```python
from build123d import *

# Parameters (mm, degrees)
SKETCH1_R             = 1.9
BOSS_EXTRUDE1_DEPTH   = 2.8
SKETCH1_R_2           = 0.8
BOSS_EXTRUDE1_2_DEPTH = 2.8
BOSS_EXTRUDE1_3_DEPTH = 2.8
SKETCH1_R_3           = 0.6
BOSS_EXTRUDE1_4_DEPTH = 2.8
BOSS_EXTRUDE1_5_DEPTH = 2.8
SKETCH2_W             = 15.494
SKETCH2_H             = 15.494
BOSS_EXTRUDE2_DEPTH   = 11.1
BOSS_EXTRUDE3_DEPTH   = 3
CHAMFER1_SIZE         = 3
CHAMFER1_SIZE2        = 5.196152423
CHAMFER1_PART_2_SIZE  = 3
CHAMFER1_PART_2_SIZE2 = 5.196152423
CHAMFER1_PART_3_SIZE  = 3
CHAMFER1_PART_3_SIZE2 = 5.196152423
CHAMFER1_PART_4_SIZE  = 3
CHAMFER1_PART_4_SIZE2 = 5.196152423
CHAMFER2_SIZE         = 4
CHAMFER2_SIZE2        = 1.455880937
CHAMFER2_PART_2_SIZE  = 4
CHAMFER2_PART_2_SIZE2 = 1.455880937
CHAMFER2_PART_3_SIZE  = 4
CHAMFER2_PART_3_SIZE2 = 1.455880937
CHAMFER2_PART_4_SIZE  = 4
CHAMFER2_PART_4_SIZE2 = 1.455880937
CHAMFER3_SIZE         = 0.5


with BuildPart() as part:
    # Sketch1 → Boss-Extrude1 (new body)
    with BuildSketch(Plane(origin=(0, 0, 0), x_dir=(1, 0, 0), z_dir=(0, 1, 0))):
        Circle(SKETCH1_R)
    extrude(amount=-BOSS_EXTRUDE1_DEPTH)



with BuildPart() as body_2:
    # Sketch1 → Boss-Extrude1 2 (new body)
    with BuildSketch(Plane(origin=(0, 0, 0), x_dir=(1, 0, 0), z_dir=(0, 1, 0))):
        with Locations((5.08, 0)):
            Circle(SKETCH1_R_2)
    extrude(amount=-BOSS_EXTRUDE1_2_DEPTH)


with BuildPart() as body_3:
    # Sketch1 → Boss-Extrude1 3 (new body)
    with BuildSketch(Plane(origin=(0, 0, 0), x_dir=(1, 0, 0), z_dir=(0, 1, 0))):
        with Locations((-5.08, 0)):
            Circle(SKETCH1_R_2)
    extrude(amount=-BOSS_EXTRUDE1_3_DEPTH)


with BuildPart() as body_4:
    # Sketch1 → Boss-Extrude1 4 (new body)
    with BuildSketch(Plane(origin=(0, 0, 0), x_dir=(1, 0, 0), z_dir=(0, 1, 0))):
        with Locations((-3.81, 2.54)):
            Circle(SKETCH1_R_3)
    extrude(amount=-BOSS_EXTRUDE1_4_DEPTH)


with BuildPart() as body_5:
    # Sketch1 → Boss-Extrude1 5 (new body)
    with BuildSketch(Plane(origin=(0, 0, 0), x_dir=(1, 0, 0), z_dir=(0, 1, 0))):
        with Locations((2.54, 5.08)):
            Circle(SKETCH1_R_3)
    extrude(amount=-BOSS_EXTRUDE1_5_DEPTH)


with BuildPart() as part_1:
    add(part.part)

    add(body_2.part)  # Boss-Extrude2 merges body 2

    add(body_3.part)  # Boss-Extrude2 merges body 3

    add(body_4.part)  # Boss-Extrude2 merges body 4

    add(body_5.part)  # Boss-Extrude2 merges body 5
    # Sketch2 → Boss-Extrude2 (add)
    with BuildSketch(Plane(origin=(0, 0, 0), x_dir=(1, 0, 0), z_dir=(0, 1, 0))):
        Rectangle(SKETCH2_W, SKETCH2_H)
    extrude(amount=BOSS_EXTRUDE2_DEPTH)

    # Sketch3 → Boss-Extrude3 (add)
    with BuildSketch(Plane(origin=(0, 11.1, 0), x_dir=(-1, 0, 0), z_dir=(0, 1, 0))):
        Polygon((0.55, -2), (-0.55, -2), (-0.55, -0.55), (-2, -0.55), (-2, 0.55), (-0.55, 0.55), (-0.55, 2), (0.55, 2), (0.55, 0.55), (2, 0.55), (2, -0.55), (0.55, -0.55), align=None)
    extrude(amount=BOSS_EXTRUDE3_DEPTH)

    # Chamfer1
    chamfer1_edges = [part_1.edges().sort_by_distance(p)[0] for p in [
        (-7.747, 11.1, 0),
    ]]
    chamfer1_side = [part_1.faces().sort_by_distance(p)[0] for p in [
        (-7.747, 5.55, 0),
    ]]
    chamfer(chamfer1_edges, length=CHAMFER1_SIZE, length2=CHAMFER1_SIZE2, reference=chamfer1_side[0])

    # Chamfer1 part 2
    chamfer1_part_2_edges = [part_1.edges().sort_by_distance(p)[0] for p in [
        (0, 11.1, 7.747),
    ]]
    chamfer1_part_2_side = [part_1.faces().sort_by_distance(p)[0] for p in [
        (0, 5.55, 7.747),
    ]]
    chamfer(chamfer1_part_2_edges, length=CHAMFER1_PART_2_SIZE, length2=CHAMFER1_PART_2_SIZE2, reference=chamfer1_part_2_side[0])

    # Chamfer1 part 3
    chamfer1_part_3_edges = [part_1.edges().sort_by_distance(p)[0] for p in [
        (7.747, 11.1, 0),
    ]]
    chamfer1_part_3_side = [part_1.faces().sort_by_distance(p)[0] for p in [
        (7.747, 5.55, 0),
    ]]
    chamfer(chamfer1_part_3_edges, length=CHAMFER1_PART_3_SIZE, length2=CHAMFER1_PART_3_SIZE2, reference=chamfer1_part_3_side[0])

    # Chamfer1 part 4
    chamfer1_part_4_edges = [part_1.edges().sort_by_distance(p)[0] for p in [
        (0, 11.1, -7.747),
    ]]
    chamfer1_part_4_side = [part_1.faces().sort_by_distance(p)[0] for p in [
        (0, 5.55, -7.747),
    ]]
    chamfer(chamfer1_part_4_edges, length=CHAMFER1_PART_4_SIZE, length2=CHAMFER1_PART_4_SIZE2, reference=chamfer1_part_4_side[0])

    # Chamfer2
    chamfer2_edges = [part_1.edges().sort_by_distance(p)[0] for p in [
        (-7.747, 0, 0),
    ]]
    chamfer2_side = [part_1.faces().sort_by_distance(p)[0] for p in [
        (-7.747, 4.05, 0),
    ]]
    chamfer(chamfer2_edges, length=CHAMFER2_SIZE, length2=CHAMFER2_SIZE2, reference=chamfer2_side[0])

    # Chamfer2 part 2
    chamfer2_part_2_edges = [part_1.edges().sort_by_distance(p)[0] for p in [
        (0, 0, 7.747),
    ]]
    chamfer2_part_2_side = [part_1.faces().sort_by_distance(p)[0] for p in [
        (0, 4.05, 7.747),
    ]]
    chamfer(chamfer2_part_2_edges, length=CHAMFER2_PART_2_SIZE, length2=CHAMFER2_PART_2_SIZE2, reference=chamfer2_part_2_side[0])

    # Chamfer2 part 3
    chamfer2_part_3_edges = [part_1.edges().sort_by_distance(p)[0] for p in [
        (7.747, 0, 0),
    ]]
    chamfer2_part_3_side = [part_1.faces().sort_by_distance(p)[0] for p in [
        (7.747, 4.05, 0),
    ]]
    chamfer(chamfer2_part_3_edges, length=CHAMFER2_PART_3_SIZE, length2=CHAMFER2_PART_3_SIZE2, reference=chamfer2_part_3_side[0])

    # Chamfer2 part 4
    chamfer2_part_4_edges = [part_1.edges().sort_by_distance(p)[0] for p in [
        (0, 0, -7.747),
    ]]
    chamfer2_part_4_side = [part_1.faces().sort_by_distance(p)[0] for p in [
        (0, 4.05, -7.747),
    ]]
    chamfer(chamfer2_part_4_edges, length=CHAMFER2_PART_4_SIZE, length2=CHAMFER2_PART_4_SIZE2, reference=chamfer2_part_4_side[0])

    # Chamfer3
    chamfer3_edges = [part_1.edges().sort_by_distance(p)[0] for p in [
        (4.28, -2.8, 0),
        (-5.88, -2.8, 0),
        (-1.9, -2.8, 0),
    ]]
    chamfer(chamfer3_edges, length=CHAMFER3_SIZE)


solid = part_1.part
```
Work out the finished part from the listing and answer in its coordinate system (mm). A direction names the side the tool comes from. Give positions to 0.01 mm unless a question says otherwise; leave off trailing zeros. Loops run counter-clockwise (first coordinate to the right, second up) from the corner with the lowest first, then second, coordinate; pieces in that order, holes last. Notation, with made-up numbers: (51, -16) - (76, -16) arc R18 ccw to (76, 4) - close; hole circle Ø6 at (0, -39). An arc over 180 degrees is marked (long way). One line per question, with ' | ' between items.
(1) The part is cut by section B-B (x = -5.08). Write down the section's boundary in (y, z), then the cut area to 3 significant figures.
Recorded:
outline: (-2.8, -0.3) - (-2.3, -0.8) - (0, -0.8) - (0, -6.29) - (4, -7.75) - (8.1, -7.75) - (9.64, -5.08) - (9.64, 5.08) - (8.1, 7.75) - (4, 7.75) - (0, 6.29) - (0, 0.8) - (-2.3, 0.8) - (-2.8, 0.3) - close | area: 144 mm²
(2) Each of these flat-tipped pins is pushed along its axis until it touches: pin 1 Ø1.6 at (y, z) = (12.5, -1) entering from -X; pin 2 Ø1.6 at (x, y) = (1, 12) entering from +Z; pin 3 Ø1.5 at (x, y) = (5.5, 3) entering from +Z. Where does it stop, or does it pass through?
Recorded:
pin 1: stops at x = -2 | pin 2: stops at z = 2 | pin 3: stops at z = 7.66
(3) The part is cut by section A-A (z = 5). Write down the section's boundary in (x, y), then the cut area to 3 significant figures.
Recorded:
outline: (-7.75, 4) - (-6.29, 0) - (6.29, 0) - (7.75, 4) - (7.75, 8.1) - (5, 9.69) - (-5, 9.69) - (-7.75, 8.1) - close | area: 140 mm²
(4) The mould has two halves that part along X. Classify faces 6 (the face through (-4.317, -1.134, -0.24)), 7 (the face through (1, 13, 0.55)), 8 (the face through (-5.69, 9.288, 0.108)): +X half, -X half, draft (parallel to the pull), parting line (faces both ways), or undercut.
Recorded:
face 6: undercut | face 7: draft | face 8: -X half
(5) A tool of negligible diameter and unlimited length cuts with its end or side. For faces 1 (the face through (0.55, 13, 1)), 2 (the face through (-2, 13, 0)), 3 (the face through (-1, 13, 0.55)), 4 (the face through (1, 13, -0.55)), 5 (the face through (-4.41, -1.38, -2.57)), from which of +Z, -Z, +X, -X, +Y, -Y can it reach the whole face along a straight path? Write none if from no direction.
Recorded:
face 1: +Z, +X, +Y | face 2: +Z, -Z, -X, +Y | face 3: +Z, -X, +Y | face 4: -Z, +X, +Y | face 5: -Y
(6) The part is cut by section C-C (y = 3). Write down the section's boundary in (x, z).
Recorded:
outline: (-7.38, -7.38) - (7.38, -7.38) - (7.38, 7.38) - (-7.38, 7.38) - close
(7) Straight lines are drawn through the part: probe 1 along Y at (x, z) = (2.25, 2.25); probe 2 along X at (y, z) = (13, -1). For each, find the intervals that lie inside material, in ascending order.
Recorded:
probe 1: y = 0 to 11.1 | probe 2: x = -0.55 to 0.55
(8) The part is cut by section D-D (z = -6). Write down the section's boundary in (x, y), then the cut area to 3 significant figures.
Recorded:
outline: (-7.75, 4) - (-6.29, 0) - (6.29, 0) - (7.75, 4) - (7.75, 8.1) - (6, 9.11) - (-6, 9.11) - (-7.75, 8.1) - close | area: 134 mm²
